Solid Edge part; units mm, degrees
sketch "Sketch1" plane through (0, 0, 0) normal (0, -1, 0) x (1, 0, 0)
  line L0 (2.5, 0) -> (2.5, 5)
  line L1 (2.5, 5) -> (7.5, 5)
  line L2 (7.5, 5) -> (7.5, 3.5)
  line L3 (7.5, 3.5) -> (6.07, 3.5)
  line L4 (6.07, 3.5) -> (6.07, 0)
  line L5 (6.07, -3.5) -> (6.07, 0)
  line L6 (7.5, -3.5) -> (6.07, -3.5)
  line L7 (7.5, -5) -> (7.5, -3.5)
  line L8 (2.5, -5) -> (7.5, -5)
  line L9 (2.5, 0) -> (2.5, -5)
  dimension "D1" = 2.5
  dimension "D2" = 6.07
revolve "RevolvedProtrusion1" add sketch "Sketch1" angle 360 about axis through (0, 0, 0) along (0, 0, 1)
properties material "Aluminum, 6061-T6"
For this review, take the finished solid that the model builds, in its own axes (mm). A direction names the side the tool comes from. Round coordinates to 2 decimals unless told otherwise and drop trailing zeros. Write each loop counter-clockwise with the first axis right and the second up, starting at its lowest first coordinate (ties: lowest second). Pieces come first, ordered by that corner, then holes. Notation, with made-up numbers: (37, 8.25) - (81, 8.25) arc R12 ccw to (81, 22.25) - close; hole circle Ø1 at (88.25, -26). An arc over 180 degrees is marked (long way). Write item = value, one per line. Start each with the question number.
1. For faces 1 (the face through (-7.493, 0.33, -4.24)), 2 (the face through (-1.316, 5.926, -0.049)), list the 3-axis set-ups (+Z, -Z, +X, -X, +Y, -Y) from which the entire face can be reached by the end or side of a thin tool; tool diameter is ignored.
2. Consider section C-C on z = -3. State the section outline as (x, y) points.
3. Consider section A-A on x = 0. State the section outline as (y, z) points.
4. For pin 1 Ø2 at (x, z) = (5.5, 3) entering from -Y; pin 2 Ø2 at (x, z) = (4, 2) entering from +Y; pin 3 Ø3 at (x, y) = (0, 0) entering from -Z, all flat-tipped, find the tip position at first contact; note any pin that passes through.
5. Draft analysis for pull direction Z (two halves, no side actions). For faces 3 (the face through (-7.493, -0.33, 4.24)), 4 (the face through (-2, 2, 5)), 5 (the face through (-2, 2, -5)), 6 (the face through (3, -6, -3.5)), state which applies: released by +Z, released by -Z, zero draft, split by the parting line, or undercut.
6. Consider section D-D on x = 4. State the section outline as (y, z) points, plus the area to 3 significant figures.
7. Wall thickness on L1, parallel to Y at x = 0, z = 0.75; L2, parallel to Z at x = 6, y = -2; L3, parallel to Y at x = 0, z = -4: over which ranges is each line inside the solid? List them lowest first.
Evaluation:
q1.face_1 = +Z, -Z
q1.face_2 = none
q2.outline = circle Ø12.14 at (0, 0); hole circle Ø5 at (0, 0)
q3.outline = (-7.5, -5) - (-2.5, -5) - (-2.5, 5) - (-7.5, 5) - (-7.5, 3.5) - (-6.07, 3.5) - (-6.07, -3.5) - (-7.5, -3.5) - close; (2.5, -5) - (7.5, -5) - (7.5, -3.5) - (6.07, -3.5) - (6.07, 3.5) - (7.5, 3.5) - (7.5, 5) - (2.5, 5) - close
q4.pin_1 = -5.9
q4.pin_2 = 5.28
q4.pin_3 = through
q5.face_3 = zero draft
q5.face_4 = released by +Z
q5.face_5 = released by -Z
q5.face_6 = undercut
q6.outline = (-6.34, -5) - (6.34, -5) - (6.34, -3.5) - (4.57, -3.5) - (4.57, 3.5) - (6.34, 3.5) - (6.34, 5) - (-6.34, 5) - (-6.34, 3.5) - (-4.57, 3.5) - (-4.57, -3.5) - (-6.34, -3.5) - close
q6.area = 102 mm2
q7.L1 = -6.07 to -2.5, 2.5 to 6.07
q7.L2 = -5 to -3.5, 3.5 to 5
q7.L3 = -7.5 to -2.5, 2.5 to 7.5
